Could you check a few things on this model? Use its own coordinates, in mm. Give positions to 0.01 mm unless a question says otherwise; leave off trailing zeros. Order: outer loops, then holes, each group sorted by start corner. A loop starts at its lowest first (then second) coordinate and runs counter-clockwise, first axis right, second up. Notation, with made-up numbers: (15, 6.5) -> (67, 6.5) arc R28 cw to (67, 45.5) -> close; hole circle Ø1 at (67, 58.5). An arc over 180 degrees is marked (long way). Write each question's results on one line, items separated by ' | '.
Autodesk Inventor part; units mm, degrees
ref_plane "YZ Plane" through (0, 0, 0) normal (1, 0, 0) x (0, 1, 0)
ref_plane "XZ Plane" through (0, 0, 0) normal (0, 1, 0) x (-1, 0, 0)
ref_plane "XY Plane" through (0, 0, 0) normal (0, 0, 1) x (1, 0, 0)
sketch "Esquisse2" plane through (0, 0, 0) normal (1, 0, 0) x (0, 1, 0)
  line L0 (0, 0) -> (0, -10.0642)
  line L1 (7.25, 2.2281) -> (7.25, 1.5734)
  line L2 (7.25, 1.5734) -> (6.55, 1.8281)
  line L3 (6.55, 1.8281) -> (6.55, 0.4)
  line L4 (6.55, 0.4) -> (7.25, 0.6548)
  line L5 (7.25, 0.6548) -> (7.25, 0)
  circle A0 centre (7.05, 1.1141) radius 0.5 construction
  line L6 (7.25, 2.2281) -> (1.5, 2.2281)
  line L7 (7.25, 0) -> (1.5, 0)
  line L8 (1.5, 0) -> (1.5, 2.2281)
  dimension "d1" = 1
  dimension "d2" = 70
  dimension "d3" = 70
  dimension "d4" = 0.2
  dimension "d5" = 14.5
  dimension "d7" = 0.4
  dimension "d8" = 0.4
  dimension "d9" = 3
revolve "Révolution1" add sketch "Esquisse2" angle 360 about axis through (0, 0, 0) along (0, 0, -1)
thread "Filetage1"
equation "\"d3\" = d2"
equation "\"d8\" = d7"
properties part number "piston_deplaceur"
Q1. I need wall thicknesses on line 1 along X through (y, z) = (0, 1.1); line 2 along X through (y, z) = (0.25, 1.9); line 3 along Z through (x, y) = (4, 6). Which ranges of each line are inside material? Lowest first, please.
Here are the results:
line 1: x = -6.55 to -1.5, 1.5 to 6.55 | line 2: x = -7.25 to -1.48, 1.48 to 7.25 | line 3: z = 0 to 0.64, 1.59 to 2.23
Q2. Suppose I cut it at C-C on z = 1.25. Please give me the cut outline in (x, y), and give its area (3 significant figures).
Here are the results:
outline: circle Ø13.1 at (0, 0); hole circle Ø3 at (0, 0) | area: 128 mm²
Q3. Thinking about a two-plate mould opening in Z: for faces 1 (the flat face through (0, 2, 2.228)), 2 (the cylindrical face through (-6.43, 3.35, 0.32)), 3 (the flat face through (0, 2, 0)), 4 (the cylindrical face through (6.494, -0.853, 1.104)), which applies, +Z half, -Z half, draft (parallel to the pull), parting line (faces both ways), or undercut?
Here are the results:
face 1: +Z half | face 2: draft | face 3: -Z half | face 4: undercut
Q4. Suppose I cut it at A-A on y = 0. Please give me the cut outline in (x, z).
Here are the results:
outline: (-7.25, 0) -> (-1.5, 0) -> (-1.5, 2.23) -> (-7.25, 2.23) -> (-7.25, 1.57) -> (-6.55, 1.83) -> (-6.55, 0.4) -> (-7.25, 0.65) -> close; (1.5, 0) -> (7.25, 0) -> (7.25, 0.65) -> (6.55, 0.4) -> (6.55, 1.83) -> (7.25, 1.57) -> (7.25, 2.23) -> (1.5, 2.23) -> close
